from build123d import *

# Parameters (mm, degrees)
SKETCH1_W           = 44.45
SKETCH1_H           = 12.7
SKETCH1_R           = 1.75
SKETCH1_W_2         = 30.48
BOSS_EXTRUDE1_DEPTH = 3.175
SKETCH2_R           = 1.75
CUT_EXTRUDE1_DEPTH  = 12.192


with BuildPart() as part:
    # Sketch1 → Boss-Extrude1 (new body)
    # profile 1 of 2: a face of its own
    with BuildSketch(Plane(origin=(0, 0, 0), x_dir=(-1, 0, 0), z_dir=(0, 1, 0))):
        Rectangle(SKETCH1_W, SKETCH1_H)
        with Locations(Location((19.05, 0, 0), (0, 0, 90))):
            Circle(SKETCH1_R, mode=Mode.SUBTRACT)
        with Locations(Location((-19.05, 0, 0), (0, 0, 90))):
            Circle(SKETCH1_R, mode=Mode.SUBTRACT)
    # profile 2 of 2: a face of its own
    with BuildSketch(Plane(origin=(0, 0, 0), x_dir=(-1, 0, 0), z_dir=(0, 1, 0))):
        with Locations((0, 12.7)):
            Rectangle(SKETCH1_W_2, SKETCH1_H)
    extrude(amount=BOSS_EXTRUDE1_DEPTH)

    # Sketch2 → Cut-Extrude1 (cut)
    with BuildSketch(Plane(origin=(0, 3.175, 0), x_dir=(-1, 0, 0), z_dir=(0, 1, 0))):
        with Locations(Location((-11.43, 12.7, 0), (0, 0, 90))):
            Circle(SKETCH2_R)
        with Locations(Location((11.43, 12.7, 0), (0, 0, 90))):
            Circle(SKETCH2_R)
    extrude(amount=-CUT_EXTRUDE1_DEPTH, mode=Mode.SUBTRACT)


solid = part.part
Work out the finished part from the listing and answer in its coordinate system (mm). A direction names the side the tool comes from. Round coordinates to 2 decimals unless told otherwise and drop trailing zeros. Write each loop counter-clockwise with the first axis right and the second up, starting at its lowest first coordinate (ties: lowest second). Pieces come first, ordered by that corner, then holes.
1) A cutting plane is placed at A-A (z = 0). Give the vertices of the cut face in (x, y) (3 decimals).
2) A tool of negligible diameter and unlimited length cuts with its end or side. For faces 4 (the flat face through (-15.24, 2, 13)), 5 (the flat face through (19, 2, 6.35)), 6 (the cylindrical face through (12.6, 1.6, 11.4)), from which of +Z, -Z, +X, -X, +Y, -Y can it reach the whole face along a straight path? Write none if from no direction.
3) The mould has two halves that part along X. Classify faces 1 (the cylindrical face through (-11.35, 1.61, 10.95)), 2 (the flat face through (0, 0, 7)), 3 (the flat face through (15.24, 2, 13)): pulls with the +X half, pulls with the -X half, needs draft (parallel to the pull), parting line crosses it, or undercut.
4) Straight lines are drawn through the part: line 1 (X direction, y = 1.4, z = 12.7); line 2 (X direction, y = 2.4, z = 0) (3 decimals); line 3 (Z direction, x = 19, y = 0.2). For each, find the intervals that lie inside material, in ascending order.
5) A cutting plane is placed at C-C (y = 1). Give the vertices of the cut face in (x, z) (3 decimals).
6) Given pin 1 Ø1 at (x, y) = (19, 1) entering from +Z; pin 2 Ø1 at (y, z) = (1.5, 15) entering from +X, each flat-ended and moving along its own axis, determine where each tip first touches the part or whether it passes through.
7) A cutting plane is placed at B-B (x = 11.43). Give the vertices of the cut face in (y, z) (3 decimals), plus the area to 3 significant figures.
8) A cutting plane is placed at D-D (x = 18.5). Give the vertices of the cut face in (y, z) (3 decimals), plus the area to 3 significant figures.
Completed:
1. outline: (-22.225, 0) - (-20.8, 0) - (-20.8, 3.175) - (-22.225, 3.175) - close; (-17.3, 0) - (17.3, 0) - (17.3, 3.175) - (-17.3, 3.175) - close; (20.8, 0) - (22.225, 0) - (22.225, 3.175) - (20.8, 3.175) - close
2. face 4: +Z, -X, +Y, -Y
2. face 5: +Z, +X, +Y, -Y
2. face 6: +Y, -Y
3. face 1: undercut
3. face 2: needs draft
3. face 3: pulls with the +X half
4. line 1: x = -15.24 to -13.18, -9.68 to 9.68, 13.18 to 15.24
4. line 2: x = -22.225 to -20.8, -17.3 to 17.3, 20.8 to 22.225
4. line 3: z = -6.35 to -1.75, 1.75 to 6.35
5. outline: (-22.225, -6.35) - (22.225, -6.35) - (22.225, 6.35) - (15.24, 6.35) - (15.24, 19.05) - (-15.24, 19.05) - (-15.24, 6.35) - (-22.225, 6.35) - close; hole circle Ø3.5 at (-19.05, 0); hole circle Ø3.5 at (-11.43, 12.7); hole circle Ø3.5 at (11.43, 12.7); hole circle Ø3.5 at (19.05, 0)
6. pin 1: stops at z = 6.35
6. pin 2: stops at x = 15.24
7. outline: (0, -6.35) - (3.175, -6.35) - (3.175, 10.95) - (0, 10.95) - close; (0, 14.45) - (3.175, 14.45) - (3.175, 19.05) - (0, 19.05) - close
7. area: 69.5 mm2
8. outline: (0, -6.35) - (3.175, -6.35) - (3.175, -1.661) - (0, -1.661) - close; (0, 1.661) - (3.175, 1.661) - (3.175, 6.35) - (0, 6.35) - close
8. area: 29.8 mm2
